from build123d import *

# Parameters (mm, degrees)
SKETCH016_R     = 3.0625
PAD003_DEPTH    = 22.5
SKETCH020_R     = 3.875
POCKET012_DEPTH = 10
SKETCH025_W     = 2.5
SKETCH025_H     = 12.25
POCKET013_DEPTH = 15
SKETCH026_W     = 2.5
SKETCH026_H     = 9.8
POCKET014_DEPTH = 9.25
SKETCH027_W     = 2.5
SKETCH027_H     = 12.25
POCKET015_DEPTH = 15
SKETCH028_W     = 2.5
SKETCH028_H     = 9.8
POCKET016_DEPTH = 9.25
SKETCH029_R     = 1.6
POCKET017_DEPTH = 5
POCKET018_DEPTH = 2


with BuildPart() as part:
    # Sketch016 → Pad003 (new body)
    with BuildSketch(Plane.XZ):
        Polygon((-56, -7), (56, -7), (56, 2), (75, 2), (75, 7), (-75, 7), (-75, 2), (-56, 2), align=None)
        with Locations((-14, 0)):
            Circle(SKETCH016_R, mode=Mode.SUBTRACT)
        with Locations((14, 0)):
            Circle(SKETCH016_R, mode=Mode.SUBTRACT)
        with Locations((-26, 0)):
            Circle(SKETCH016_R, mode=Mode.SUBTRACT)
        with Locations((26, 0)):
            Circle(SKETCH016_R, mode=Mode.SUBTRACT)
    extrude(amount=PAD003_DEPTH)

    # Sketch020 (on Face4 of Pad003) → Pocket012 (cut)
    with BuildSketch(Plane(origin=(0, 0, -7), x_dir=(1, 0, 0), z_dir=(0, 0, -1))):
        with Locations((-44.75, 11.25)):
            Circle(SKETCH020_R)
        with Locations((44.75, 11.3)):
            Circle(SKETCH020_R)
    extrude(amount=-POCKET012_DEPTH, mode=Mode.SUBTRACT)

    # Sketch025 (on Face9 of Pocket012) → Pocket013 (cut)
    with BuildSketch(Plane(origin=(56, 0, 0), x_dir=(0, 0, 1), z_dir=(1, 0, 0))):
        with Locations((-0.75, 6.125)):
            Rectangle(SKETCH025_W, SKETCH025_H)
    extrude(amount=-POCKET013_DEPTH, mode=Mode.SUBTRACT)

    # Sketch026 (on Face11 of Pocket013) → Pocket014 (cut)
    with BuildSketch(Plane(origin=(41, 0, 0), x_dir=(0, 0, 1), z_dir=(1, 0, 0))):
        with Locations((-0.75, 7.35)):
            Rectangle(SKETCH026_W, SKETCH026_H)
    extrude(amount=-POCKET014_DEPTH, mode=Mode.SUBTRACT)

    # Sketch027 (on Face7 of Pocket012) → Pocket015 (cut)
    with BuildSketch(Plane(origin=(-56, 0, 0), x_dir=(0, 0, -1), z_dir=(-1, 0, 0))):
        with Locations((0.75, 6.125)):
            Rectangle(SKETCH027_W, SKETCH027_H)
    extrude(amount=-POCKET015_DEPTH, mode=Mode.SUBTRACT)

    # Sketch028 (on Face9 of Pocket015) → Pocket016 (cut)
    with BuildSketch(Plane(origin=(-41, 0, 0), x_dir=(0, 0, -1), z_dir=(-1, 0, 0))):
        with Locations((0.75, 7.35)):
            Rectangle(SKETCH028_W, SKETCH028_H)
    extrude(amount=-POCKET016_DEPTH, mode=Mode.SUBTRACT)

    # Sketch029 (on Face2 of Pocket016) → Pocket017 (cut)
    with BuildSketch(Plane(origin=(0, 0, 7), x_dir=(-1, 0, 0), z_dir=(0, 0, 1))):
        with Locations((-66.75, 11.25)):
            Circle(SKETCH029_R)
        with Locations((66.75, 11.25)):
            Circle(SKETCH029_R)
    extrude(amount=-POCKET017_DEPTH, mode=Mode.SUBTRACT)

    # Sketch030 (on Face18 of Pocket017) → Pocket018 (cut)
    with BuildSketch(Plane(origin=(0, 0, 2), x_dir=(1, 0, 0), z_dir=(0, 0, -1))):
        Polygon((-65.125, 8.4354174377), (-63.5, 11.25), (-65.125, 14.0645825623), (-68.375, 14.0645825623), (-70, 11.25), (-68.375, 8.4354174377), align=None)
        Polygon((68.375, 8.4354174377), (70, 11.25), (68.375, 14.0645825623), (65.125, 14.0645825623), (63.5, 11.25), (65.125, 8.4354174377), align=None)
    extrude(amount=-POCKET018_DEPTH, mode=Mode.SUBTRACT)


solid = part.part
Could you check a few things on this model? Use its own coordinates, in mm. A direction names the side the tool comes from. Coordinates: 2 decimals unless noted, no trailing zeros. Order: outer loops, then holes, each group sorted by start corner. A loop starts at its lowest first (then second) coordinate and runs counter-clockwise, first axis right, second up.
Q1. Suppose I cut it at C-C on y = -19.5. Please give me the cut outline in (x, z) (1 decimal).
Q2. Thinking about a two-plate mould opening in Z: for faces 1 (the flat face through (-36, -2.45, -1)), 2 (the flat face through (75, -11, 4)), 3 (the flat face through (-44, -6, 0.5)), 4 (the flat face through (65, -12, 4)), which applies, released by +Z, released by -Z, zero draft, split by the parting line, or undercut?
Q3. Please list where these lines run through material, in increasing order: L1, parallel to X at y = -11.3, z = -3.25 (3 decimals); L2, parallel to Z at x = -32.5, y = -11.75; L3, parallel to X at y = -13, z = -6.5.
Q4. Which directions (+Z, -Z, +X, -X, +Y, -Y) give clear straight access to the entire face, cutting with the end or side of a thin tool? Please do faces 5 (the flat face through (31.75, -7, -1)), 6 (the cylindrical face through (-45.254, -15.092, -2.07)), 7 (the flat face through (-44, -6, -2)).
Q5. Will these pins go through, and if not, where does the flat tip stop? pin 1 (1 mm diameter, centred on y = -13, z = -5.5, fed in from +X); pin 2 (3 mm diameter, centred on y = -9.5, z = -0.5, fed in from -X); pin 3 (6 mm diameter, centred on x = -67.5, y = -11.5, fed in from -Z).
Q6. Suppose I cut it at B-B on x = -33.5. Please give me the cut outline in (y, z), and give its area (4 significant figures).
Q7. Suppose I cut it at D-D on x = 53.5. Please give me the cut outline in (y, z), and give its area (3 significant figures).
Q8. Suppose I cut it at A-A on x = -66.75. Please give me the cut outline in (y, z), and give its area (3 significant figures).
Answer:
1. outline: (-75, 2) - (-56, 2) - (-56, -7) - (56, -7) - (56, 2) - (75, 2) - (75, 7) - (-75, 7) - close; hole circle Ø6.1 at (-26, 0); hole circle Ø6.1 at (-14, 0); hole circle Ø6.1 at (14, 0); hole circle Ø6.1 at (26, 0)
2. face 1: undercut
2. face 2: zero draft
2. face 3: undercut
2. face 4: released by -Z
3. L1: x = -56 to -48.625, -40.875 to 40.875, 48.625 to 56
3. L2: z = -7 to -2, 0.5 to 7
3. L3: x = -56 to -48.21, -41.29 to 41.27, 48.23 to 56
4. face 5: +X
4. face 6: -Z
4. face 7: -X
5. pin 1: stops at x = 56
5. pin 2: stops at x = -56
5. pin 3: stops at z = 2
6. outline: (-22.5, -7) - (0, -7) - (0, 7) - (-22.5, 7) - close; hole (-12.25, -2) - (-2.45, -2) - (-2.45, 0.5) - (-12.25, 0.5) - close
6. area: 290.5 mm2
7. outline: (-22.5, -7) - (0, -7) - (0, -2) - (-12.25, -2) - (-12.25, 0.5) - (0, 0.5) - (0, 7) - (-22.5, 7) - close
7. area: 284 mm2
8. outline: (-22.5, 2) - (-14.06, 2) - (-14.06, 4) - (-12.85, 4) - (-12.85, 7) - (-22.5, 7) - close; (-9.65, 4) - (-8.44, 4) - (-8.44, 2) - (0, 2) - (0, 7) - (-9.65, 7) - close
8. area: 91.6 mm2
